```python
from build123d import *

# Parameters (mm, degrees)
SKETCH1_R           = 62.5
BOSS_EXTRUDE1_DEPTH = 6
CUT_EXTRUDE1_START  = 55
SKETCH2_R           = 2
CUT_EXTRUDE1_DEPTH  = 13
CUT_EXTRUDE2_START  = -68
SKETCH2_2_R         = 2
CUT_EXTRUDE2_DEPTH  = 13
CUT_EXTRUDE3_START  = 55
SKETCH3_R           = 2
CUT_EXTRUDE3_DEPTH  = 13
CUT_EXTRUDE4_START  = -68
SKETCH3_2_R         = 2
CUT_EXTRUDE4_DEPTH  = 13
BOSS_EXTRUDE2_START = 12
BOSS_EXTRUDE2_DEPTH = 12
FILLET1_R           = 10
CUT_EXTRUDE8_START  = 60
SKETCH6_R           = 2
CUT_EXTRUDE8_DEPTH  = 12.5
CHAMFER1_SIZE       = 1


with BuildPart() as part:
    # Sketch1 → Boss-Extrude1 (new, symmetric)
    with BuildSketch(Plane.XY):
        Circle(SKETCH1_R)
    extrude(amount=BOSS_EXTRUDE1_DEPTH, both=True)

    # Sketch2 → Cut-Extrude1 (cut)
    with BuildSketch(Plane(origin=(0, 0, 0), x_dir=(1, 0, 0), z_dir=(0, 1, 0)).offset(CUT_EXTRUDE1_START)):
        with Locations(Location((0, 0, 0), (0, 0, 90))):
            Circle(SKETCH2_R)
    extrude(amount=CUT_EXTRUDE1_DEPTH, mode=Mode.SUBTRACT)

    # Sketch2_2 → Cut-Extrude2 (cut)
    with BuildSketch(Plane(origin=(0, 0, 0), x_dir=(1, 0, 0), z_dir=(0, 1, 0)).offset(CUT_EXTRUDE2_START)):
        with Locations(Location((0, 0, 0), (0, 0, 90))):
            Circle(SKETCH2_2_R)
    extrude(amount=CUT_EXTRUDE2_DEPTH, mode=Mode.SUBTRACT)

    # Sketch3 → Cut-Extrude3 (cut)
    with BuildSketch(Plane(origin=(0, 0, 0), x_dir=(0, 0, -1), z_dir=(1, 0, 0)).offset(CUT_EXTRUDE3_START)):
        Circle(SKETCH3_R)
    extrude(amount=CUT_EXTRUDE3_DEPTH, mode=Mode.SUBTRACT)

    # Sketch3_2 → Cut-Extrude4 (cut)
    with BuildSketch(Plane(origin=(0, 0, 0), x_dir=(0, 0, -1), z_dir=(1, 0, 0)).offset(CUT_EXTRUDE4_START)):
        Circle(SKETCH3_2_R)
    extrude(amount=CUT_EXTRUDE4_DEPTH, mode=Mode.SUBTRACT)

    # Sketch5 → Boss-Extrude2 (add)
    with BuildSketch(Plane.XY.offset(6).offset(BOSS_EXTRUDE2_START)):
        with BuildLine():
            Line((-31.25, 54.126587737), (-28.75, 49.796460718))
            ThreePointArc((-28.75, 49.796460718), (0, 57.5), (28.75, 49.796460718))
            Line((28.75, 49.796460718), (31.25, 54.126587737))
            ThreePointArc((31.25, 54.126587737), (0, 62.5), (-31.25, 54.126587737))
        make_face()
    extrude(amount=-BOSS_EXTRUDE2_DEPTH)

    # Fillet1
    fillet1_edges = [part.edges().sort_by_distance(p)[0] for p in [
        (-30, 51.961524227, 18),
        (30, 51.961524227, 18),
    ]]
    fillet(fillet1_edges, radius=FILLET1_R)

    # Sketch6 → Cut-Extrude8 (cut)
    with BuildSketch(Plane(origin=(0, 0, 0), x_dir=(1, 0, 0), z_dir=(0, 1, 0)).offset(CUT_EXTRUDE8_START)):
        with Locations(Location((0, -12, 0), (0, 0, 90))):
            Circle(SKETCH6_R)
    extrude(amount=CUT_EXTRUDE8_DEPTH, mode=Mode.SUBTRACT)

    # Chamfer1
    chamfer1_edges = [part.edges().sort_by_distance(p)[0] for p in [
        (-62.5, 0, -6),
    ]]
    chamfer(chamfer1_edges, length=CHAMFER1_SIZE)


solid = part.part
```
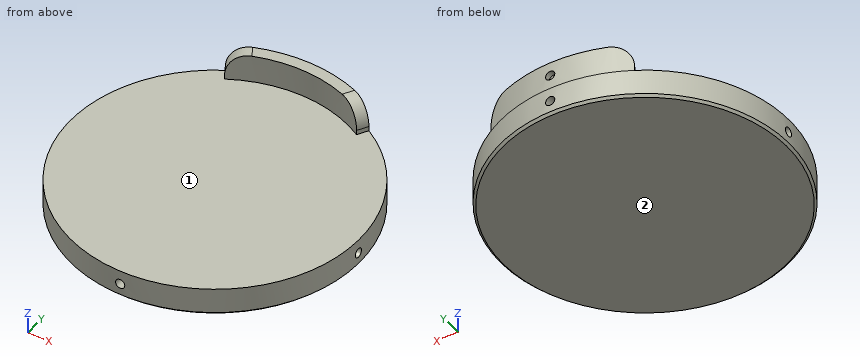
Geometry check sheet. Reference: the model listing, model coordinates, mm. Face numbers are marked on the shaded views. Coordinates: 2 decimals unless noted, no trailing zeros. Loops run counter-clockwise (first coordinate to the right, second up) from the corner with the lowest first, then second, coordinate; pieces in that order, holes last.
Item 1: Release check for a two-part mould opening along Z. For the marked faces 1 and 2 record: released by +Z, released by -Z, zero draft, split by the parting line, or undercut.
Item 2: Sectioned sample at B-B, the plane x = 0. Record the boundary of the cut face in (y, z), then the cut area to 3 significant figures.
Item 3: Thickness scan on line 1 (Z direction, x = -58, y = 0); line 2 (Z direction, x = -20.5, y = 35.5); line 3 (Y direction, x = 55.5, z = 5.75). Record the ranges inside material, lowest first.
Item 4: Sectioned sample at C-C, the plane z = 12. Record the boundary of the cut face in (x, y).
Item 5: Go/stop test with flat-tipped pins: pin 1 Ø1.2 at (y, z) = (-1, 0) entering from +X; pin 2 Ø6 at (x, y) = (14.5, 11) entering from +Z; pin 3 Ø12 at (x, z) = (-46, 15) entering from +Y; pin 4 Ø6 at (y, z) = (-39, -1.5) entering from -X. Record where each tip stops, or that it passes through.
Item 6: Sectioned sample at A-A, the plane y = 0. Record the boundary of the cut face in (x, z), then the cut area to 3 significant figures.
Item 7: Sectioned sample at D-D, the plane z = 0. Record the boundary of the cut face in (x, y), then the cut area to 3 significant figures.
Check result:
1. face 1: released by +Z
1. face 2: released by -Z
2. outline: (-62.5, -5) - (-61.5, -6) - (61.5, -6) - (62.5, -5) - (62.5, -2) - (55, -2) - (55, 2) - (62.5, 2) - (62.5, 10) - (60, 10) - (60, 14) - (62.5, 14) - (62.5, 18) - (57.5, 18) - (57.5, 6) - (-62.5, 6) - (-62.5, 2) - (-55, 2) - (-55, -2) - (-62.5, -2) - close
2. area: 1,490 mm2
3. line 1: z = -6 to -2, 2 to 6
3. line 2: z = -6 to 6
3. line 3: y = -28.74 to 28.74
4. outline: (-30.52, 54.54) - (-28.02, 50.21) arc R57.5 cw to (28.02, 50.21) - (30.52, 54.54) arc R62.5 ccw to (2, 62.47) - (2, 60) - (-2, 60) - (-2, 62.47) arc R62.5 ccw to start
5. pin 1: stops at x = 55
5. pin 2: stops at z = 6
5. pin 3: passes through
5. pin 4: stops at x = -51.09
6. outline: (-62.5, -5) - (-61.5, -6) - (61.5, -6) - (62.5, -5) - (62.5, -2) - (55, -2) - (55, 2) - (62.5, 2) - (62.5, 6) - (-62.5, 6) - (-62.5, 2) - (-55, 2) - (-55, -2) - (-62.5, -2) - close
6. area: 1,440 mm2
7. outline: (-62.47, -2) arc R62.5 ccw to (-2, -62.47) - (-2, -55) - (2, -55) - (2, -62.47) arc R62.5 ccw to (62.47, -2) - (55, -2) - (55, 2) - (62.47, 2) arc R62.5 ccw to (2, 62.47) - (2, 55) - (-2, 55) - (-2, 62.47) arc R62.5 ccw to (-62.47, 2) - (-55, 2) - (-55, -2) - close
7. area: 12,200 mm2
